Solid Edge part; units mm, degrees
sketch "Sketch1" plane through (0, 0, 0) normal (0, 0, 1) x (1, 0, 0)
  circle A0 centre (0, 0) radius 12.5
extrude "Protrusion1" add sketch "Sketch1" along normal blind 3
sketch "Sketch2" plane through (0, 0, 3) normal (0, 0, 1) x (1, 0, 0)
  circle A0 centre (0, 0) radius 10
extrude "ProtrusioneEstrusa_2" add sketch "Sketch2" along normal blind 3
sketch "Sketch3" plane through (0, 0, 6) normal (0, 0, 1) x (1, 0, 0)
  circle A0 centre (0, 0) radius 5
extrude "Cutout1" cut sketch "Sketch3" against normal through all
Geometry check sheet. Reference: the model listing, model coordinates, mm. A direction names the side the tool comes from. Give positions to 0.01 mm unless a question says otherwise; leave off trailing zeros. Write each loop counter-clockwise with the first axis right and the second up, starting at its lowest first coordinate (ties: lowest second). Pieces come first, ordered by that corner, then holes. Notation, with made-up numbers: (17.5, -23.75) - (76.5, -23.75) arc R21 ccw to (76.5, 5.25) - close; hole circle Ø1 at (22, 89.5). An arc over 180 degrees is marked (long way). Use a Markdown table: item, result.
Q1. Thickness scan on L1, parallel to Y at x = 0, z = 1.45; L2, parallel to Y at x = 0, z = 4.05; L3, parallel to Z at x = 9.5, y = -6. Record the ranges inside material, lowest first. Write a range as [from, to].
Computed:
| item | result |
|---|---|
| L1 | y = [-12.5, -5], [5, 12.5] |
| L2 | y = [-10, -5], [5, 10] |
| L3 | z = [0, 3] |
Q2. Draft check along X on faces 1 (the face through (-1.08, -4.88, 3.04)), 2 (the face through (-2.17, 9.76, 4.48)), 3 (the face through (-0.2, -5.4, 0)). Enter one of: pulls with the +X half, pulls with the -X half, needs draft (parallel to the pull), parting line crosses it, or undercut.
Computed:
| item | result |
|---|---|
| face 1 | undercut |
| face 2 | parting line crosses it |
| face 3 | needs draft |
Q3. Set-up check for faces 4 (the face through (-0.1, 10.2, 3)), 5 (the face through (11.923, -3.755, 1.479)): record each of +Z, -Z, +X, -X, +Y, -Y from which the full face is reachable in a straight line by a thin tool's end or side.
Computed:
| item | result |
|---|---|
| face 4 | +Z |
| face 5 | +Z, -Z |
Q4. Section check D-D, the plane x = -7.25. Enter the section's corners in (y, z).
Computed:
| item | result |
|---|---|
| outline | (-10.18, 0) - (10.18, 0) - (10.18, 3) - (6.89, 3) - (6.89, 6) - (-6.89, 6) - (-6.89, 3) - (-10.18, 3) - close |
Q5. Go/stop test with flat-tipped pins: P1, Ø2, axis at x = 5, z = 3.5, coming from the -Y side; P2, Ø1, axis at y = -3.5, z = 5.5, coming from the +X side; P3, Ø3, axis at y = -6.5, z = 1.5, coming from the +X side. Record where each tip stops, or that it passes through.
Computed:
| item | result |
|---|---|
| P1 | stops at y = -11.8 |
| P2 | stops at x = 9.54 |
| P3 | stops at x = 11.46 |
Q6. Section check C-C, the plane z = 0.75. Enter the section's corners in (x, y), then the cut area to 3 significant figures.
Computed:
| item | result |
|---|---|
| outline | circle Ø25 at (0, 0); hole circle Ø10 at (0, 0) |
| area | 412 mm² |
Q7. Section check A-A, the plane x = 0. Enter the section's corners in (y, z).
Computed:
| item | result |
|---|---|
| outline | (-12.5, 0) - (-5, 0) - (-5, 6) - (-10, 6) - (-10, 3) - (-12.5, 3) - close; (5, 0) - (12.5, 0) - (12.5, 3) - (10, 3) - (10, 6) - (5, 6) - close |
